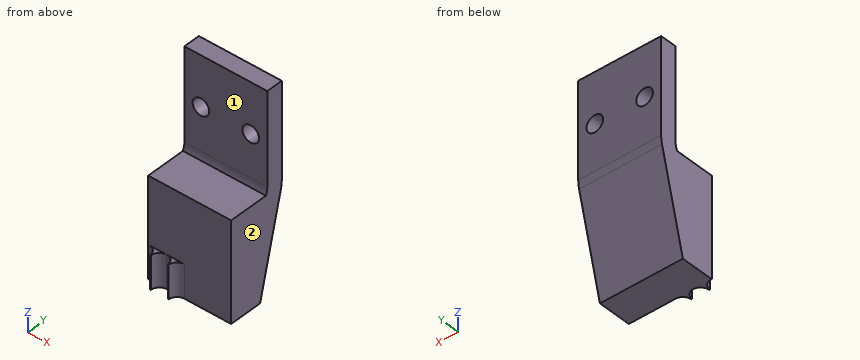
from build123d import *

# Parameters (mm, degrees)
SKETCH1_W           = 60
SKETCH1_H           = 20
SKETCH1_H_2         = 10
BOSS_EXTRUDE1_DEPTH = 50
FILLET1_R           = 20
BOSS_EXTRUDE2_DEPTH = 50
FILLET2_R           = 10
BOSS_EXTRUDE3_DEPTH = 20
FILLET3_R           = 5
SKETCH4_R           = 5
CUT_EXTRUDE1_DEPTH  = 10


with BuildPart() as part:
    # Sketch1 → Boss-Extrude1 (new body)
    with BuildSketch(Plane(origin=(0, 0, 0), x_dir=(0, 0, -1), z_dir=(1, 0, 0))):
        Rectangle(SKETCH1_W, SKETCH1_H)
        Polygon((-30, 25), (30, 10), (-30, 10), align=None)
        with Locations((-60, 20)):
            Rectangle(SKETCH1_W, SKETCH1_H_2)
    extrude(amount=BOSS_EXTRUDE1_DEPTH)

    # Fillet1
    fillet1_edges = [part.edges().sort_by_distance(p)[0] for p in [
        (25, 25, 30),
    ]]
    fillet(fillet1_edges, radius=FILLET1_R)

    # Sketch2 → Boss-Extrude2 (add)
    with BuildSketch(Plane.ZY):
        Polygon((30, 15), (30, 14), (31, 15), align=None)
    extrude(amount=-BOSS_EXTRUDE2_DEPTH)

    # Fillet2
    # the kernel refuses this fillet: 10 mm, written as the material it adds along each edge
    with BuildSketch(Plane(origin=(0, 15, 31), x_dir=(0, 0, 1), z_dir=(1, 0, 0))) as fillet2_piece_1:
        with BuildLine():
            CenterArc((3.358898944, 10), FILLET2_R, 244.158067237, 25.841932763)
            Line((-1, 1), (-1.087177979, 0.82))
            ThreePointArc((-1.087177979, 0.82), (-0.641421356, 0.358578644), (-0.141421356, -0.141421356))
            Line((-0.141421356, -0.141421356), (0, -0.2))
            Line((0, -0.2), (3.358898944, -0.2))
            Line((3.358898944, -0.2), (3.358898944, 0))
        make_face()
    extrude(amount=50)

    # Sketch3 → Boss-Extrude3 (add)
    with BuildSketch(Plane(origin=(0, 0, -30), x_dir=(-1, 0, 0), z_dir=(0, 0, -1))):
        with BuildLine():
            Line((-5.55, -10), (-11.149999969, -10))
            ThreePointArc((-11.149999969, -10), (-7.543755405, -11.493755427), (-6.05, -15.1))
            Line((-6.05, -15.1), (-5.55, -15.1))
            Line((-5.55, -15.1), (-5.55, -10))
        make_face()
        with BuildLine():
            Line((-16.75, -15.1), (-16.25, -15.1))
            ThreePointArc((-16.25, -15.1), (-14.756244573, -11.493755405), (-11.149999969, -10))
            Line((-11.149999969, -10), (-16.75, -10))
            Line((-16.75, -10), (-16.75, -15.1))
        make_face()
    extrude(amount=-BOSS_EXTRUDE3_DEPTH)

    # Fillet3
    fillet3_edges = [part.edges().sort_by_distance(p)[0] for p in [
        (5.55, -10, -20),
        (16.75, -10, -20),
    ]]
    fillet(fillet3_edges, radius=FILLET3_R)

    # Sketch4 → Cut-Extrude1 (cut)
    with BuildSketch(Plane(origin=(0, 25, 0), x_dir=(1, 0, 0), z_dir=(0, 1, 0))):
        with Locations(Location((10, -60, 0), (0, 0, 270))):
            Circle(SKETCH4_R)
        with Locations(Location((40, -60, 0), (0, 0, 270))):
            Circle(SKETCH4_R)
    extrude(amount=-CUT_EXTRUDE1_DEPTH, mode=Mode.SUBTRACT)


solid = part.part
Work out the finished part from the listing and answer in its coordinate system (mm). Face numbers are marked on the shaded views. A direction names the side the tool comes from. Round coordinates to 2 decimals unless told otherwise and drop trailing zeros. Loops run counter-clockwise (first coordinate to the right, second up) from the corner with the lowest first, then second, coordinate; pieces in that order, holes last. Notation, with made-up numbers: (77, 68) -> (109, 68) arc R34 ccw to (109, 98) -> close; hole circle Ø2 at (-5.75, 32). An arc over 180 degrees is marked (long way). Use one line per item in the form item = value.
(1) Find section A-A on z = 60. Give the vertices of the cut face in (x, y), then the cut area to 3 significant figures.
Answer list:
outline = (0, 15) -> (5, 15) -> (5, 25) -> (0, 25) -> close; (15, 15) -> (35, 15) -> (35, 25) -> (15, 25) -> close; (45, 15) -> (50, 15) -> (50, 25) -> (45, 25) -> close
area = 300 mm2
(2) Flat-ended cylindrical pins translate along their axes: P1, Ø6, axis at x = 27, z = -5.5, coming from the +Y side (3 decimals); P2, Ø5.5, axis at x = 6, y = -12.5, coming from the +Z side; P3, Ø1.5, axis at y = 11.5, z = 27.5, coming from the -X side; P4, Ø1.5, axis at y = 14, z = 47, coming from the -X side. Find the tip coordinate at first contact, or state that the pin passes through.
Answer list:
P1 = 16.875
P2 = 30
P3 = 0
P4 = through
(3) Straight lines are drawn through the part: line 1 (X direction, y = 20, z = 60); line 2 (Z direction, x = 35, y = -4.5); line 3 (Y direction, x = 5, z = 79.5). For each, find the intervals that lie inside material, in ascending order.
Answer list:
line_1 = 0 to 5, 15 to 35, 45 to 50
line_2 = -30 to 30
line_3 = 15 to 25
(4) Find section B-B on x = 37. Give the vertices of the cut face in (y, z), then the cut area to 3 significant figures.
Answer list:
outline = (-10, -30) -> (10, -30) -> (24.4, 27.61) arc R20 ccw to (25, 32.46) -> (25, 56) -> (15, 56) -> (15, 34.36) arc R10 cw to (14, 30) -> (-10, 30) -> close; (15, 64) -> (25, 64) -> (25, 90) -> (15, 90) -> close
area = 2,170 mm2
(5) A tool of negligible diameter and unlimited length cuts with its end or side. For the marked faces 1 and 2, from which of +Z, -Z, +X, -X, +Y, -Y can it reach the whole face along a straight path? Write none if from no direction.
Answer list:
face_1 = +Z, +X, -X, -Y
face_2 = +Z, -Z, +X, +Y, -Y
(6) Find section C-C on x = 10. Give the vertices of the cut face in (y, z), then the cut area to 3 significant figures.
Answer list:
outline = (-10.13, -30) -> (10, -30) -> (24.4, 27.61) arc R20 ccw to (25, 32.46) -> (25, 55) -> (15, 55) -> (15, 34.36) arc R10 cw to (14, 30) -> (-10, 30) -> (-10, -10) -> (-10.13, -10) -> close; (15, 65) -> (25, 65) -> (25, 90) -> (15, 90) -> close
area = 2,150 mm2
(7) Find section D-D on z = 38.5. Give the vertices of the cut face in (x, y).
Answer list:
outline = (0, 15) -> (50, 15) -> (50, 25) -> (0, 25) -> close
